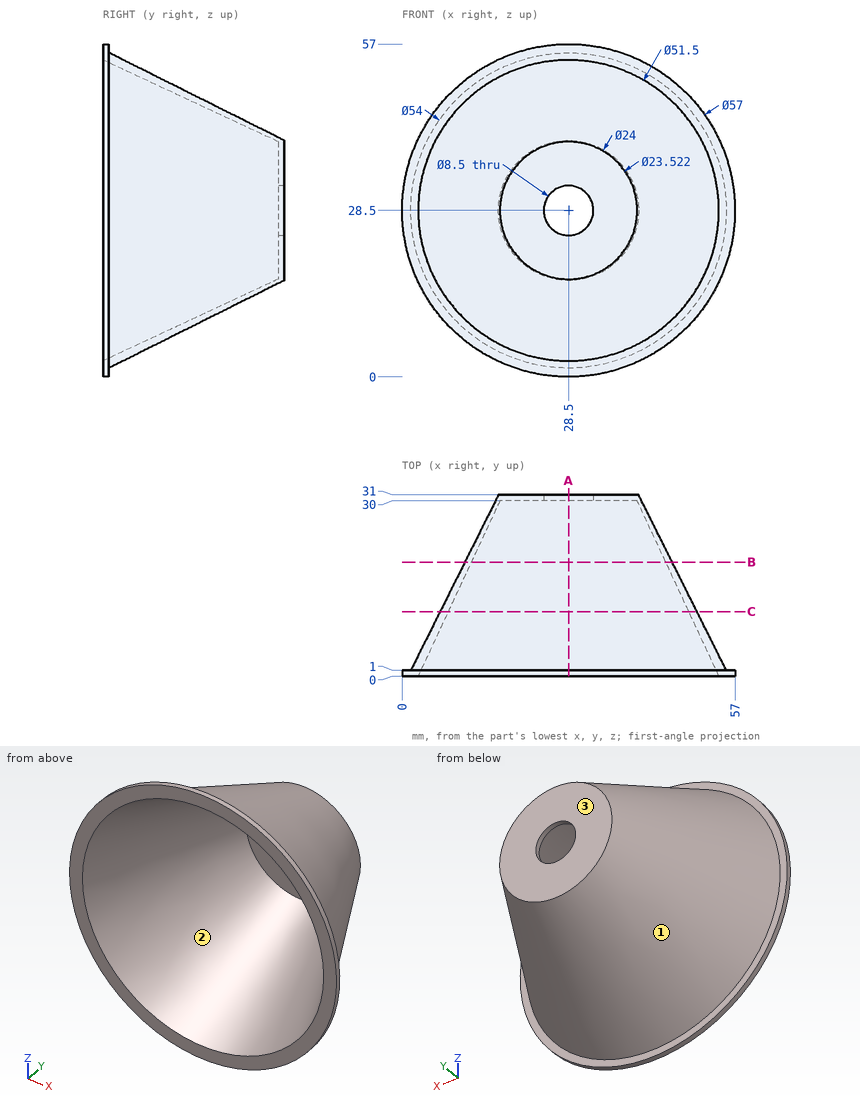
Verification items for this drawing (mm, ordinates from the low corner). Give positions to 0.01 mm unless a question says otherwise; leave off trailing zeros. Write each loop counter-clockwise with the first axis right and the second up, starting at its lowest first coordinate (ties: lowest second). Pieces come first, ordered by that corner, then holes. Notation, with made-up numbers: (67, -25.75) -> (101, -25.75) arc R18 ccw to (101, 1.25) -> close; hole circle Ø8 at (52.5, -1). An arc over 180 degrees is marked (long way). Use CSV: the item, a comma, the result in double quotes. Start each with the question number.
Q1. Release check for a two-part mould opening along Z. For the marked faces 1, 2 and 3 record: +Z half, -Z half, draft (parallel to the pull), parting line (faces both ways), or undercut.
Q2. Scan lines: line 1 along Y through (x, z) = (36, 23); line 2 along Y through (x, z) = (52.5, 42); line 3 along X through (y, z) = (10, 13) (1 decimal). Record each from-to range of solid material in increasing order.
Q3. Depth check by flat-ended pin: P1, Ø2, axis at y = 6.5, z = 32.5, coming from the +X side; P2, Ø4, axis at x = 8, y = 9.5, coming from the +Z side (1 decimal); P3, Ø10, axis at x = 14.5, y = 7, coming from the -Z side (1 decimal). Enter the tip coordinate at first touch or a pass-through.
Q4. Cross-section at C-C on y = 11. Enter the section's corners in (x, z).
Q5. Cross-section at A-A on x = 28.5. Enter the section's corners in (y, z).
Q6. Cross-section at B-B on y = 19.5. Enter the section's corners in (x, z), and give its area (3 significant figures).
Working result:
1,face 1,"parting line"
1,face 2,"undercut"
1,face 3,"draft"
2,line 1,"y = 30 to 31"
2,line 2,"y = 0 to 1"
2,line 3,"x = 12.2 to 14.2, 42.8 to 44.8"
3,P1,"stops at x = 52.95"
3,P2,"stops at z = 42.2"
3,P3,"stops at z = 4.9"
4,outline,"circle Ø44 at (28.5, 28.5); hole circle Ø41.24 at (28.5, 28.5)"
5,outline,"(0, 0) -> (1, 0) -> (1, 1.5) -> (31, 16.5) -> (31, 24.25) -> (30, 24.25) -> (30, 16.74) -> (0, 2.75) -> close; (0, 54.25) -> (30, 40.26) -> (30, 32.75) -> (31, 32.75) -> (31, 40.5) -> (1, 55.5) -> (1, 57) -> (0, 57) -> close"
6,outline,"circle Ø35.5 at (28.5, 28.5); hole circle Ø33.31 at (28.5, 28.5)"
6,area,"118 mm^2"
